Check sheet for the modelled part. Datum: model origin and axes. Units: mm. A direction names the side the tool comes from. Round coordinates to 2 decimals unless told otherwise and drop trailing zeros. Order: outer loops, then holes, each group sorted by start corner. A loop starts at its lowest first (then second) coordinate and runs counter-clockwise, first axis right, second up.
Q1. Scan lines: probe 1 along X at (y, z) = (30, -0.9); probe 2 along X at (y, z) = (28, -1.55); probe 3 along Y at (x, z) = (83, -0.75). Record each from-to range of solid material in increasing order.
Q2. Set-up check for faces 1 (the cylindrical face through (84.077, 8.069, -2.555)), 2 (the cylindrical face through (64.268, 10.909, -0.986)), 3 (the flat face through (85.751, -1, -2)), 4 (the flat face through (85.751, 36, -2)): record each of +Z, -Z, +X, -X, +Y, -Y from which the full face is reachable in a straight line by a thin tool's end or side.
Q3. Mould release check, pull along X, two halves, no side actions. Record for faces 5 (the cylindrical face through (45.448, -4.224, -1.541)), 6 (the cylindrical face through (58.392, 40.227, -1.584)), 7 (the flat face through (64, 6, -2)): +X half, -X half, draft (parallel to the pull), parting line (faces both ways), or undercut.
Q4. Cross-section at B-B on y = 33. Record the cut outline in (x, z) (3 decimals).
Q5. Cross-section at C-C on x = 53.5. Record the cut outline in (y, z) (3 decimals).
Q6. Cross-section at D-D on z = -0.95. Give the number of separate pieces and of enclosed holes in the cut face, then the cut area to 3 significant figures.
Q7. Cross-section at A-A on x = 63.5. Record the cut outline in (y, z) (1 decimal).
Q8. Depth check by flat-ended pin: P1, Ø1, axis at y = 11.5, z = -2, coming from the +X side; P2, Ø1.5, axis at y = 12.5, z = -2, coming from the -X side; P3, Ø6.5, axis at x = 62.5, y = 7.5, coming from the +Z side. Enter the tip coordinate at first touch or a pass-through.
from build123d import *

# Parameters (mm, degrees)
MODEL_R             = 3.875
MODEL_R_2           = 2.7
MODEL_R_3           = 2.125
BOSS_EXTRUDE1_DEPTH = 3.125
MODEL_3_R           = 4.125
MODEL_3_R_2         = 2.125
CUT_EXTRUDE1_DEPTH  = 2
FILLET1_R           = 3
FILLET2_R           = 6


with BuildPart() as part:
    # Model → Boss-Extrude1 (new body)
    with BuildSketch(Plane.XY):
        with BuildLine():
            Line((57.940219492, 39.930508181), (85.751165458, 39.930508181))
            Line((85.751165458, 39.930508181), (85.751165458, 34.091112415))
            ThreePointArc((85.751165458, 34.091112415), (87.9590359, 28.077103201), (93.457436342, 24.789156838))
            ThreePointArc((93.457436342, 24.789156838), (99.50819863, 17.430508181), (93.457436342, 10.071859524))
            ThreePointArc((93.457436342, 10.071859524), (87.9590359, 6.783913161), (85.751165458, 0.769903947))
            Line((85.751165458, 0.769903947), (85.751165458, -5.069491819))
            Line((85.751165458, -5.069491819), (57.940219492, -5.069491819))
            ThreePointArc((57.940219492, -5.069491819), (45.846452894, -4.78733661), (48.573590158, 6.998312478))
            ThreePointArc((48.573590158, 6.998312478), (55.686625956, 17.430508181), (48.573590158, 27.862703884))
            ThreePointArc((48.573590158, 27.862703884), (45.846452894, 39.648352972), (57.940219492, 39.930508181))
        make_face()
        with Locations((92.00819863, 17.430508181)):
            Circle(MODEL_R, mode=Mode.SUBTRACT)
        with Locations((52.008207521, -0.004787091)):
            Circle(MODEL_R_2, mode=Mode.SUBTRACT)
        with Locations((52.008207521, 34.865803453)):
            Circle(MODEL_R_2, mode=Mode.SUBTRACT)
        with Locations((82.050054867, 7.430508181)):
            Circle(MODEL_R_3, mode=Mode.SUBTRACT)
        with Locations((62.05010788, 7.430508181)):
            Circle(MODEL_R_3, mode=Mode.SUBTRACT)
        with Locations((82.050054867, 27.430508181)):
            Circle(MODEL_R_3, mode=Mode.SUBTRACT)
        with Locations((62.05010788, 27.430508181)):
            Circle(MODEL_R_3, mode=Mode.SUBTRACT)
    extrude(amount=-BOSS_EXTRUDE1_DEPTH)

    # Model_3 → Cut-Extrude1 (cut)
    with BuildSketch(Plane.XY):
        with Locations((82.050054867, 7.430508181)):
            Circle(MODEL_3_R)
        with Locations((82.050054867, 7.430508181)):
            Circle(MODEL_3_R_2, mode=Mode.SUBTRACT)
        with Locations((62.05010788, 7.430508181)):
            Circle(MODEL_3_R)
        with Locations((62.05010788, 7.430508181)):
            Circle(MODEL_3_R_2, mode=Mode.SUBTRACT)
        with Locations((62.05010788, 27.430508181)):
            Circle(MODEL_3_R)
        with Locations((62.05010788, 27.430508181)):
            Circle(MODEL_3_R_2, mode=Mode.SUBTRACT)
        with Locations((82.050054867, 27.430508181)):
            Circle(MODEL_3_R)
    extrude(amount=-CUT_EXTRUDE1_DEPTH, mode=Mode.SUBTRACT)

    # Fillet1
    fillet1_edges = [part.edges().sort_by_distance(p)[0] for p in [
        (85.751165458, 39.930508181, -1.5625),
        (85.751165458, -5.069491819, -1.5625),
    ]]
    fillet(fillet1_edges, radius=FILLET1_R)

    # Fillet2
    fillet2_edges = [part.edges().sort_by_distance(p)[0] for p in [
        (57.940219492, 39.930508181, -1.5625),
        (57.940219492, -5.069491819, -1.5625),
    ]]
    fillet(fillet2_edges, radius=FILLET2_R)


solid = part.part
Results found:
1. probe 1: x = 45.91 to 58.82, 65.28 to 78.82, 85.28 to 86.72
1. probe 2: x = 48.31 to 57.96, 66.14 to 77.96, 86.14 to 88.02
1. probe 3: y = -5.06 to 3.42, 11.44 to 23.42, 31.44 to 39.92
2. face 1: +Z, -Z
2. face 2: +Z
2. face 3: +Z, -Z, +X, -Y
2. face 4: +Z, -Z, +X, +Y
3. face 5: parting line
3. face 6: +X half
3. face 7: undercut
4. outline: (44.435, -3.125) - (50.057, -3.125) - (50.057, 0) - (44.435, 0) - close; (53.96, -3.125) - (85.826, -3.125) - (85.826, 0) - (53.96, 0) - close
5. outline: (-7.661, -3.125) - (-2.255, -3.125) - (-2.255, 0) - (-7.661, 0) - close; (2.246, -3.125) - (10.78, -3.125) - (10.78, 0) - (2.246, 0) - close; (24.081, -3.125) - (32.615, -3.125) - (32.615, 0) - (24.081, 0) - close; (37.116, -3.125) - (42.522, -3.125) - (42.522, 0) - (37.116, 0) - close
6. separate pieces: 1
6. enclosed holes: 7
6. area: 1,600 mm2
7. outline: (-5.1, -3.1) - (5.9, -3.1) - (5.9, -2) - (3.6, -2) - (3.6, 0) - (-5.1, 0) - close; (9, -3.1) - (25.9, -3.1) - (25.9, -2) - (23.6, -2) - (23.6, 0) - (11.3, 0) - (11.3, -2) - (9, -2) - close; (29, -3.1) - (39.9, -3.1) - (39.9, 0) - (31.3, 0) - (31.3, -2) - (29, -2) - close
8. P1: stops at x = 97.18
8. P2: stops at x = 54.14
8. P3: stops at z = -2
